Source: CAD feature listing. Evaluate the final solid. Frame: model axes, mm. A direction names the side the tool comes from. Give positions to 0.01 mm unless a question says otherwise; leave off trailing zeros. Order: outer loops, then holes, each group sorted by start corner. A loop starts at its lowest first (then second) coordinate and runs counter-clockwise, first axis right, second up. Notation, with made-up numbers: (51.25, -28) - (66.25, -28) arc R22 cw to (66.25, -1) - close; hole circle Ø10 at (-14, -26.5). An arc over 180 degrees is marked (long way). Answer as CSV lines item,"result".
```python
from build123d import *

# Parameters (mm, degrees)
FILETE1_R = 0.4
FILETE2_R = 0.4
FILETE3_R = 0.4


with BuildPart() as part:
    # Esboço1 → Revolução1 (revolve)
    with BuildSketch(Plane.XY, mode=Mode.PRIVATE) as revolu_o1_sk:
        with BuildLine():
            Line((0, 0), (0, 5.55))
            Line((0, 5.55), (1.4, 5.55))
            Line((1.4, 5.55), (1.4, 4.8))
            Line((1.4, 4.8), (33, 4.8))
            Line((33, 4.8), (33, 4.6))
            Line((33, 4.6), (34, 4.6))
            Line((34, 4.6), (40, 3))
            Line((40, 3), (40, 1.5))
            ThreePointArc((40, 1.5), (38.939339828, 1.060660172), (38.5, 0))
            Line((38.5, 0), (0, 0))
        make_face()
    revolve(revolu_o1_sk.sketch.rotate(Axis((38.5, 0, 0), (-1, 0, 0)), 90), axis=Axis((38.5, 0, 0), (-1, 0, 0)))

    # Filete1
    # the kernel refuses this fillet: 0.4 mm, written as the material it takes off along each edge
    with BuildSketch(Plane(origin=(33, 0, 0), x_dir=(0, 0, -1), z_dir=(0, 1, 0))) as filete1_piece_1:
        with BuildLine():
            CenterArc((4.4, 0.346410162), FILETE1_R, 300, 60)
            Line((4.6, 0), (4.604, -0.006928203))
            ThreePointArc((4.604, -0.006928203), (4.7, -0.008), (4.8, -0.008))
            Line((4.8, -0.008), (4.808, 0))
            Line((4.808, 0), (4.808, 0.346410162))
            Line((4.808, 0.346410162), (4.8, 0.346410162))
        make_face()
    revolve(axis=Axis((33, 0, 0), (-1, 0, 0)), mode=Mode.SUBTRACT)

    # Filete2
    filete2_edges = [part.edges().sort_by_distance(p)[0] for p in [
        (34, 0, 4.6),
    ]]
    fillet(filete2_edges, radius=FILETE2_R)

    # Filete3
    filete3_edges = [part.edges().sort_by_distance(p)[0] for p in [
        (40, 0, 3),
    ]]
    fillet(filete3_edges, radius=FILETE3_R)


solid = part.part
```
(1) Contact query for flat-ended pins moving along their axis: pin 1 (4 mm diameter, centred on x = 9.5, z = 0, fed in from -Y); pin 2 (2 mm diameter, centred on x = 22.5, y = 1.5, fed in from +Z); pin 3 (1 mm diameter, centred on y = 2, z = -2.5, fed in from -X); pin 4 (3 mm diameter, centred on x = 30, y = 3.5, fed in from -Z). Output: stop coordinate, or through.
Completed:
pin 1,"y = -4.8"
pin 2,"z = 4.77"
pin 3,"x = 0"
pin 4,"z = -4.36"
(2) Ray query, line 1 (X direction, y = 5.25, z = 0.5); line 2 (Z direction, x = 3.5, y = 0); line 3 (X direction, y = -2.75, z = -1). Return the intervals inside material, ascending. Write a range as from..to.
Completed:
line 1,"0..1.4"
line 2,"-4.8..4.8"
line 3,"0..39.92"
(3) Cut plane A-A (x = 28). Return loops of the section in (y, z).
Completed:
outline,"circle Ø9.6 at (0, 0)"
(4) Access query for faces 1 (the flat face through (40, 1.2, -1.2)), 2 (the cylindrical face through (33.48, 4.49, 1)). Directions: +Z, -Z, +X, -X, +Y, -Y. A direction counts if a zero-diameter tool reaches every point of the face in a straight line with its end or side. Return the directions, or none.
Completed:
face 1,"+Z, -Z, +X, +Y, -Y"
face 2,"+X"
